```python
from build123d import *

# Parameters (mm, degrees)
SKETCH1_W           = 53.6
SKETCH1_H           = 40.64
SKETCH1_W_2         = 11.3
BOSS_EXTRUDE1_DEPTH = 76.2
SHELL1_T            = -6.35
SKETCH2_W           = 20
SKETCH2_H           = 40.9
SKETCH2_R           = 2
CUT_EXTRUDE1_DEPTH  = 116.171565935
SKETCH3_R           = 3.175
BOSS_EXTRUDE2_DEPTH = 10
FILLET2_R           = 2.54
CUT_EXTRUDE2_REACH  = 121.068
SKETCH5_W           = 12.7
SKETCH5_H           = 6.35


with BuildPart() as part:
    # Sketch1 → Boss-Extrude1 (new body)
    with BuildSketch(Plane.XY):
        with Locations((38.1, 20.32)):
            Rectangle(SKETCH1_W, SKETCH1_H)
        with Locations((5.65, 20.32)):
            Rectangle(SKETCH1_W_2, SKETCH1_H)
        with Locations((70.55, 20.32)):
            Rectangle(SKETCH1_W_2, SKETCH1_H)
    extrude(amount=BOSS_EXTRUDE1_DEPTH)

    # Shell1
    shell1_openings = [part.faces().sort_by_distance(p)[0] for p in [
        (38.1, 0, 38.1),
    ]]
    offset(amount=SHELL1_T, openings=shell1_openings, kind=Kind.INTERSECTION)

    # Sketch2 → Cut-Extrude1 (cut, through all)
    with BuildSketch(Plane(origin=(0, 40.64, 0), x_dir=(1, 0, 0), z_dir=(0, 1, 0))):
        with Locations((38.1, -38.1)):
            Rectangle(SKETCH2_W, SKETCH2_H)
        with Locations(Location((43.1, -62.4, 0), (0, 0, 270))):
            Circle(SKETCH2_R)
        with Locations(Location((33.1, -62.4, 0), (0, 0, 270))):
            Circle(SKETCH2_R)
        with Locations(Location((33.1, -13.8, 0), (0, 0, 270))):
            Circle(SKETCH2_R)
        with Locations(Location((43.1, -13.8, 0), (0, 0, 270))):
            Circle(SKETCH2_R)
    extrude(amount=-CUT_EXTRUDE1_DEPTH, mode=Mode.SUBTRACT)

    # Sketch3 → Boss-Extrude2 (add)
    with BuildSketch(Plane(origin=(0, 40.64, 0), x_dir=(1, 0, 0), z_dir=(0, 1, 0))):
        with Locations(Location((15.875, -27.65044, 0), (0, 0, 270))):
            Circle(SKETCH3_R)
        with Locations(Location((60.325, -27.65044, 0), (0, 0, 270))):
            Circle(SKETCH3_R)
    extrude(amount=BOSS_EXTRUDE2_DEPTH)

    # Fillet2
    fillet2_edges = [part.edges().sort_by_distance(p)[0] for p in [
        (15.875, 50.64, 24.47544),
        (60.325, 50.64, 24.47544),
    ]]
    fillet(fillet2_edges, radius=FILLET2_R)

    # Sketch5 → Cut-Extrude2 (cut, up to next)
    with BuildSketch(Plane(origin=(0, 0, 0), x_dir=(-1, 0, 0), z_dir=(0, 0, -1)), mode=Mode.PRIVATE) as cut_extrude2_sk1:
        with Locations((-38.1, 3.175)):
            Rectangle(SKETCH5_W, SKETCH5_H)
    cut_extrude2_tool1 = extrude(cut_extrude2_sk1.sketch, amount=-CUT_EXTRUDE2_REACH, mode=Mode.PRIVATE) & part.part
    add(cut_extrude2_tool1.solids().sort_by_distance((38.1, 3.175, 0))[0], mode=Mode.SUBTRACT)


solid = part.part
```
Input: part model. Units: mm. Frame: model coordinates. A direction names the side the tool comes from. Round coordinates to 2 decimals unless told otherwise and drop trailing zeros. Loops run counter-clockwise (first coordinate to the right, second up) from the corner with the lowest first, then second, coordinate; pieces in that order, holes last. Notation, with made-up numbers: (36, -8.75) -> (86, -8.75) arc R22 ccw to (86, 21.25) -> close; hole circle Ø4 at (-4, 8.5). An arc over 180 degrees is marked (long way). Use one line per item in the form item = value. Start each with the question number.
Item 1: Material intervals for L1, parallel to X at y = 39.25, z = 13.8; L2, parallel to Z at x = 43, y = 38; L3, parallel to Z at x = 31, y = 21, sorted ascending. Write a range as from..to.
Item 2: Section query B-B on x = 33.1. Return the cut outline in (y, z), then the cut area to 3 significant figures.
Item 3: Mould query, pull axis Z, two halves, no side actions, for faces 5 (the face through (44.45, 3, 3)), 6 (the face through (38, 21, 76.2)), 7 (the face through (63, 44.32, 29.36)), 8 (the face through (31.9, 37.5, 12.2)). Classes: pulls with the +Z half, pulls with the -Z half, needs draft (parallel to the pull), parting line crosses it, or undercut.
Item 4: Set-up query: faces 1 (the face through (76.2, 20, 38)), 2 (the face through (38, 6.35, 3)), 3 (the face through (48.1, 38, 38)), 4 (the face through (6.35, 17, 38)). Return all of +Z, -Z, +X, -X, +Y, -Y with unobstructed straight access to the full face (end or side cutting, diameter ignored); none if empty.
Item 5: Section query A-A on z = 37. Return the cut outline in (x, y).
Item 6: Section query D-D on z = 62.4. Return the cut outline in (x, y).
Item 7: Section query C-C on y = 29. Return the cut outline in (x, z), then the cut area to 3 significant figures.
Item 8: Contact query for flat-ended pins moving along their axis: pin 1 Ø2 at (x, z) = (53, 12.5) entering from +Y; pin 2 Ø7 at (x, z) = (39.5, 4) entering from -Y; pin 3 Ø3 at (y, z) = (4.5, 2) entering from -X; pin 4 Ø3 at (x, z) = (47, 47) entering from -Y. Output: stop coordinate, or through.
Ans:
q1.L1 = 0..31.1, 35.1..41.1, 45.1..76.2
q1.L2 = 0..11.8, 15.8..17.65, 58.55..60.4, 64.4..76.2
q1.L3 = 0..6.35, 69.85..76.2
q2.outline = (0, 69.85) -> (34.29, 69.85) -> (34.29, 64.4) -> (40.64, 64.4) -> (40.64, 76.2) -> (0, 76.2) -> close; (6.35, 0) -> (40.64, 0) -> (40.64, 11.8) -> (34.29, 11.8) -> (34.29, 6.35) -> (6.35, 6.35) -> close; (34.29, 15.8) -> (40.64, 15.8) -> (40.64, 17.65) -> (34.29, 17.65) -> close; (34.29, 58.55) -> (40.64, 58.55) -> (40.64, 60.4) -> (34.29, 60.4) -> close
q2.area = 569 mm^2
q3.face_5 = needs draft
q3.face_6 = pulls with the +Z half
q3.face_7 = parting line crosses it
q3.face_8 = undercut
q4.face_1 = +Z, -Z, +X, +Y, -Y
q4.face_2 = -Z, -Y
q4.face_3 = +Y, -Y
q4.face_4 = -Y
q5.outline = (0, 0) -> (6.35, 0) -> (6.35, 34.29) -> (28.1, 34.29) -> (28.1, 40.64) -> (0, 40.64) -> close; (48.1, 34.29) -> (69.85, 34.29) -> (69.85, 0) -> (76.2, 0) -> (76.2, 40.64) -> (48.1, 40.64) -> close
q6.outline = (0, 0) -> (6.35, 0) -> (6.35, 34.29) -> (31.1, 34.29) -> (31.1, 40.64) -> (0, 40.64) -> close; (35.1, 34.29) -> (41.1, 34.29) -> (41.1, 40.64) -> (35.1, 40.64) -> close; (45.1, 34.29) -> (69.85, 34.29) -> (69.85, 0) -> (76.2, 0) -> (76.2, 40.64) -> (45.1, 40.64) -> close
q7.outline = (0, 0) -> (76.2, 0) -> (76.2, 76.2) -> (0, 76.2) -> close; hole (6.35, 6.35) -> (69.85, 6.35) -> (69.85, 69.85) -> (6.35, 69.85) -> close
q7.area = 1,770 mm^2
q8.pin_1 = 40.64
q8.pin_2 = 6.35
q8.pin_3 = 0
q8.pin_4 = 34.29
